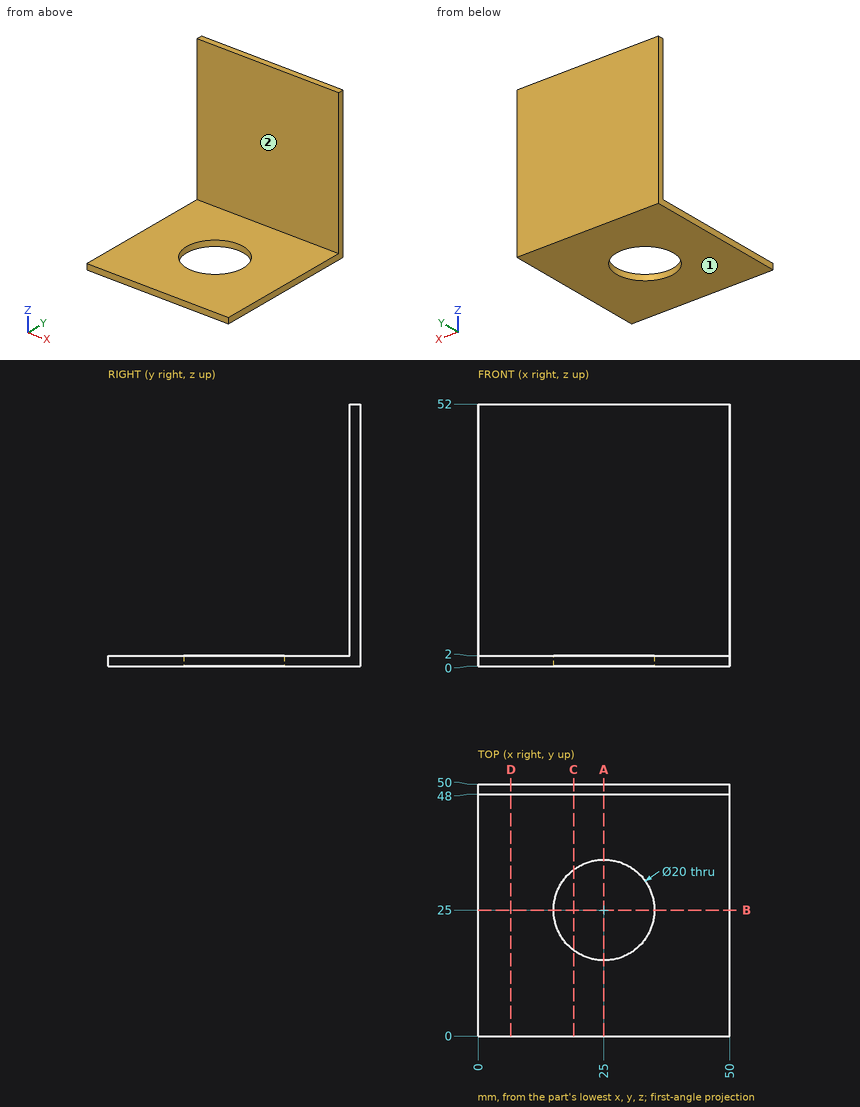
Answer from the drawing. Dimensions are ordinates in mm from the lowest x, y and z of the part. A direction names the side the tool comes from. Give positions to 0.01 mm unless a question says otherwise; leave off trailing zeros. Loops run counter-clockwise (first coordinate to the right, second up) from the corner with the lowest first, then second, coordinate; pieces in that order, holes last. Notation, with made-up numbers: M 48,37.25 L 105,37.25 A31 cw 105,62.25 Z; hole C 56,-40 d10. An arc over 180 degrees is marked long. One line per item, written item: value.
Q1. A cutting plane is placed at A-A on x = 25. Determine the outline of the cut face in (y, z), then the cut area to 3 significant figures.
Working result:
outline: M 0,0 L 15,0 L 15,2 L 0,2 Z; M 35,0 L 50,0 L 50,52 L 48,52 L 48,2 L 35,2 Z
area: 160 mm^2
Q2. A flat-ended cylindrical pin translates along its axis: P1, Ø8, axis at x = 30, z = 19, coming from the -Y side. Find the tip coordinate at first contact, or state that the pin passes through.
Working result:
P1: stops at y = 48
Q3. A cutting plane is placed at B-B on y = 25. Determine the outline of the cut face in (x, z).
Working result:
outline: M 0,0 L 15,0 L 15,2 L 0,2 Z; M 35,0 L 50,0 L 50,2 L 35,2 Z
Q4. A cutting plane is placed at C-C on x = 19. Determine the outline of the cut face in (y, z), then the cut area to 3 significant figures.
Working result:
outline: M 0,0 L 17,0 L 17,2 L 0,2 Z; M 33,0 L 50,0 L 50,52 L 48,52 L 48,2 L 33,2 Z
area: 168 mm^2
Q5. A cutting plane is placed at D-D on x = 6.5. Determine the outline of the cut face in (y, z), then the cut area to 3 significant figures.
Working result:
outline: M 0,0 L 50,0 L 50,52 L 48,52 L 48,2 L 0,2 Z
area: 200 mm^2
Q6. Find the intervals of material crossed by line 1 (Y direction, x = 25, z = 1); line 2 (Y direction, x = 25.5, z = 37); line 3 (Z direction, x = 8.5, y = 20.5), in increasing order. Write a range as from..to.
Working result:
line 1: y = 0..15, 35..50
line 2: y = 48..50
line 3: z = 0..2
Q7. For the marked faces 1 and 2, determine the directions among +Z, -Z, +X, -X, +Y, -Y from which every point of the face is accessible in a straight line to the end or side of a thin tool.
Working result:
face 1: -Z, +X, -X, +Y, -Y
face 2: +Z, +X, -X, -Y
